For this review, take the finished solid that the model builds, in its own axes (mm). Face numbers are marked on the shaded views. A direction names the side the tool comes from. Coordinates: 2 decimals unless noted, no trailing zeros. Write each loop counter-clockwise with the first axis right and the second up, starting at its lowest first coordinate (ties: lowest second). Pieces come first, ordered by that corner, then holes. Notation, with made-up numbers: M 12.25,73 L 63.25,73 A22 cw 63.25,85 Z; hole C 43.25,82.5 d9. An arc over 180 degrees is marked long. One line per question, with ' | ' between items.
from build123d import *

# Parameters (mm, degrees)
SKETCH_1_W      = 9
SKETCH_1_H      = 4
EXTRUDE_1_DEPTH = 55


with BuildPart() as part:
    # Эскиз1 → Бобышка-Вытянуть1 (new body)
    with BuildSketch(Plane(origin=(0, 0, 0), x_dir=(1, 0, 0), z_dir=(0, 1, 0))):
        with BuildLine():
            ThreePointArc((6.5, 0), (4.596194078, 4.596194078), (0, 6.5))
            Line((0, 6.5), (0, 4))
            ThreePointArc((0, 4), (2.828427125, 2.828427125), (4, 0))
            ThreePointArc((4, 0), (3.464101615, -2), (2, -3.464101615))
            Line((2, -3.464101615), (2, -6.184658438))
            ThreePointArc((2, -6.184658438), (5.25594901, -3.824264635), (6.5, 0))
        make_face()
        with BuildLine():
            Line((0, -4), (0, -6.5))
            ThreePointArc((0, -6.5), (1.01235373, -6.420680643), (2, -6.184658438))
            Line((2, -6.184658438), (2, -3.464101615))
            ThreePointArc((2, -3.464101615), (1.03527618, -3.863703305), (0, -4))
        make_face()
        with BuildLine():
            ThreePointArc((2, -6.184658438), (1.01235373, -6.420680643), (0, -6.5))
            Line((0, -6.5), (0, -17))
            Line((0, -17), (2, -17))
            Line((2, -17), (2, -13))
            Line((2, -13), (2, -6.184658438))
        make_face()
        with Locations((6.5, -15)):
            Rectangle(SKETCH_1_W, SKETCH_1_H)
    extrude(amount=EXTRUDE_1_DEPTH)

    # Зеркальное отражение1: part across plane


with BuildPart() as part_1:
    add(part.part)
    add(part.part.mirror(Plane(origin=(0, 55, 0), x_dir=(0, 0, 1), z_dir=(1, 0, 0))))


solid = part_1.part
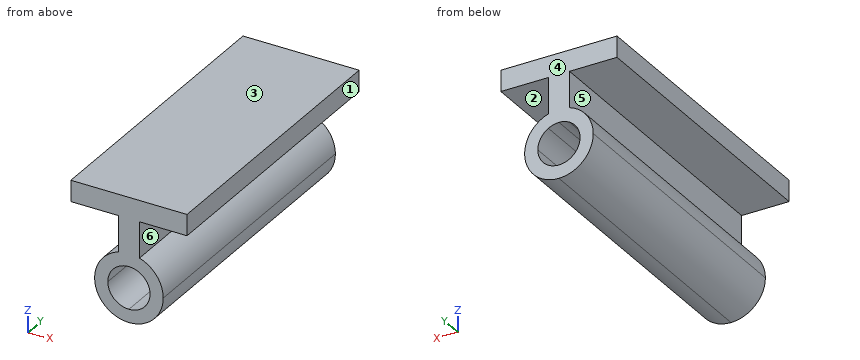
1) To check wall thickness, follow line 1 along Z through (x, y) = (-0.25, 42); line 2 along X through (y, z) = (21, 0); line 3 along Z through (x, y) = (-3.25, 36). State the ranges of each line that lie inside material, in increasing order. Write a range as [from, to].
Responses:
line 1: [-6.5, -3.99], [3.99, 17] | line 2: [-6.5, -4], [4, 6.5] | line 3: [-5.63, -2.33], [2.33, 5.63], [13, 17]
2) Machinability: for the marked faces 4, 5 and 6, which of the approach directions +Z, -Z, +X, -X, +Y, -Y give a long, thin tool a straight path to every point of the face, cutting with its end or side? Answer none if there is none.
Responses:
face 4: +Z, -Z, +X, -X, +Y | face 5: -X, +Y, -Y | face 6: +X, +Y, -Y
3) The part is to be moulded in two halves that separate along Z. For the marked faces 1, 2 and 3, say which applies: +Z half, -Z half, draft (parallel to the pull), parting line (faces both ways), or undercut.
Responses:
face 1: draft | face 2: undercut | face 3: +Z half
4) We need section A-A on x = 5.25. State the section outline as (y, z) points, then the cut area to 3 significant figures.
Responses:
outline: M 0,-3.83 L 55,-3.83 L 55,3.83 L 0,3.83 Z; M 0,13 L 55,13 L 55,17 L 0,17 Z | area: 642 mm^2
5) We need section B-B on y = 10. State the section outline as (x, z) points, then the cut area to 3 significant figures.
Responses:
outline: M -11,13 L -2,13 L -2,6.18 A6.5 ccw long 2,6.18 L 2,13 L 11,13 L 11,17 L -11,17 Z; hole C 0,0 d8 | area: 197 mm^2
6) We need section C-C on z = -1.5. State the section outline as (x, y) points, then the cut area to 3 significant figures.
Responses:
outline: M -6.32,0 L -3.71,0 L -3.71,55 L -6.32,55 Z; M 3.71,0 L 6.32,0 L 6.32,55 L 3.71,55 Z | area: 288 mm^2
7) We need section D-D on x = 9.5. State the section outline as (y, z) points.
Responses:
outline: M 0,13 L 55,13 L 55,17 L 0,17 Z
8) Insertion check: pin 1 Ø2 at (y, z) = (25, 8.5) entering from +X; pin 2 Ø1.5 at (y, z) = (14.5, 9.5) entering from -X; pin 3 Ø4.5 at (x, y) = (-4.5, 29.5) entering from -Z. Each pin has a flat end and moves straight along its axis. Give the tip position at first contact, or say it passes through.
Responses:
pin 1: x = 2 | pin 2: x = -2 | pin 3: z = -6.1
